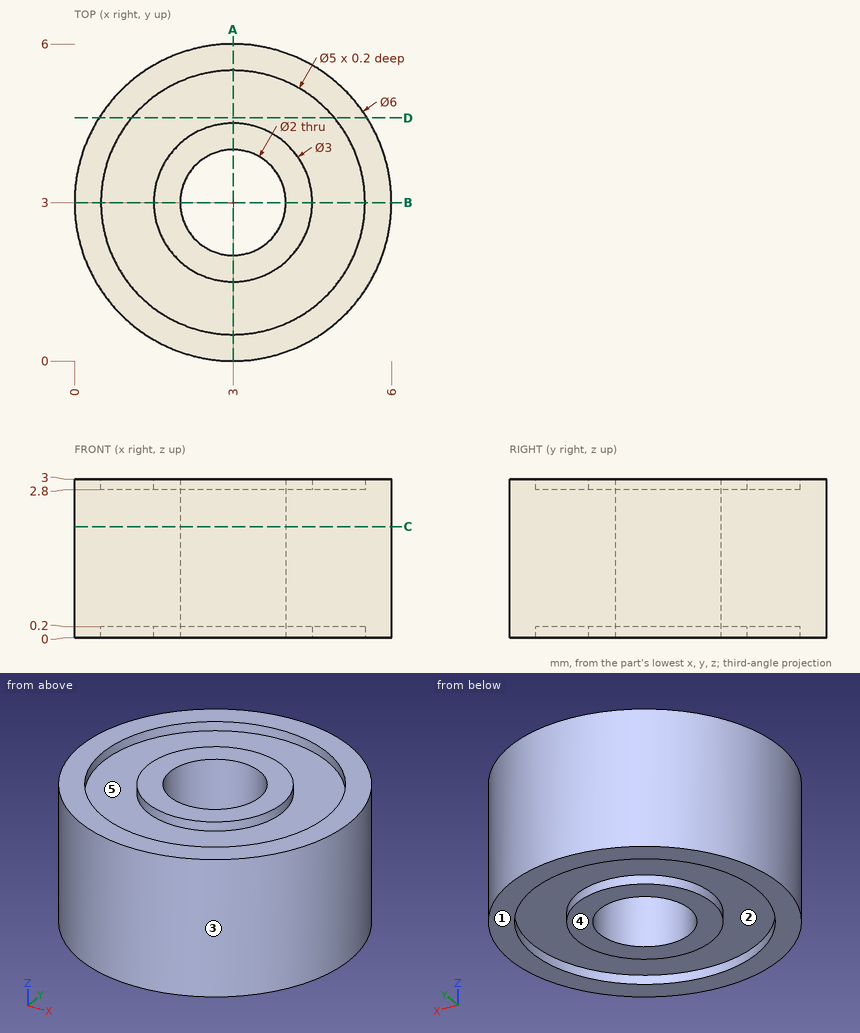
Here's the drawing with two shaded views (mm, measured from the low corner). I have some questions. A direction names the side the tool comes from. Give positions to 0.01 mm unless a question says otherwise; leave off trailing zeros. Loops run counter-clockwise (first coordinate to the right, second up) from the corner with the lowest first, then second, coordinate; pieces in that order, holes last. Notation, with made-up numbers: M 25,76 L 58,76 A7 ccw 58,83 Z; hole C 48.5,36 d1. An arc over 180 degrees is marked long. Answer in a Markdown table with one row per item.
1. Suppose I cut it at C-C on z = 2.1. Write out the boundary of the cut face in (x, y), plus the area to 3 significant figures.
Taken from the geometry:
| item | result |
|---|---|
| outline | C 3,3 d6; hole C 3,3 d2 |
| area | 25.1 mm² |
2. For pin 1 Ø3 at (x, y) = (3, 3) entering from +Z; pin 2 Ø1.5 at (y, z) = (4, 1.5) entering from -X, each with a flat end and sliding along its axis, tell me the tip position at first contact or that it passes through.
Taken from the geometry:
| item | result |
|---|---|
| pin 1 | stops at z = 3 |
| pin 2 | stops at x = 0.01 |
3. If I drill on line 1 along Y through (x, z) = (3, 0.15); line 2 along Z through (x, y) = (1.5, 3.4); line 3 along Y through (x, z) = (3, 1.6), over which ranges is the centre line in solid material (lowest first)?
Taken from the geometry:
| item | result |
|---|---|
| line 1 | y = 0 to 0.5, 1.5 to 2, 4 to 4.5, 5.5 to 6 |
| line 2 | z = 0.2 to 2.8 |
| line 3 | y = 0 to 2, 4 to 6 |
4. Suppose I cut it at A-A on x = 3. Write out the boundary of the cut face in (y, z), plus the area to 3 significant figures.
Taken from the geometry:
| item | result |
|---|---|
| outline | M 0,0 L 0.5,0 L 0.5,0.2 L 1.5,0.2 L 1.5,0 L 2,0 L 2,3 L 1.5,3 L 1.5,2.8 L 0.5,2.8 L 0.5,3 L 0,3 Z; M 4,0 L 4.5,0 L 4.5,0.2 L 5.5,0.2 L 5.5,0 L 6,0 L 6,3 L 5.5,3 L 5.5,2.8 L 4.5,2.8 L 4.5,3 L 4,3 Z |
| area | 11.2 mm² |
5. Thinking about a two-plate mould opening in X: for the marked faces 3, 4 and 5, which applies, released by +X, released by -X, zero draft, split by the parting line, or undercut?
Taken from the geometry:
| item | result |
|---|---|
| face 3 | split by the parting line |
| face 4 | zero draft |
| face 5 | undercut |
6. Suppose I cut it at D-D on y = 4.6. Write out the boundary of the cut face in (x, z), plus the area to 3 significant figures.
Taken from the geometry:
| item | result |
|---|---|
| outline | M 0.46,0 L 1.08,0 L 1.08,0.2 L 4.92,0.2 L 4.92,0 L 5.54,0 L 5.54,3 L 4.92,3 L 4.92,2.8 L 1.08,2.8 L 1.08,3 L 0.46,3 Z |
| area | 13.7 mm² |
7. Which directions (+Z, -Z, +X, -X, +Y, -Y) give clear straight access to the entire face, cutting with the end or side of a thin tool? Please do the marked faces 1 and 2.
Taken from the geometry:
| item | result |
|---|---|
| face 1 | -Z, +X, -X, +Y, -Y |
| face 2 | -Z |
